Build history of the part. All positions in model axes, mm. Face numbers are marked on the shaded views. A direction names the side the tool comes from. Round coordinates to 2 decimals unless told otherwise and drop trailing zeros. Write each loop counter-clockwise with the first axis right and the second up, starting at its lowest first coordinate (ties: lowest second). Pieces come first, ordered by that corner, then holes. Notation, with made-up numbers: (66.25, 29) -> (123.25, 29) arc R33 ccw to (123.25, 68) -> close; hole circle Ø6 at (73.25, -26.75). An arc over 180 degrees is marked (long way). One line per question, with ' | ' between items.
from build123d import *

# Parameters (mm, degrees)
SKETCH1_W           = 60
SKETCH1_H           = 25
BOSS_EXTRUDE1_DEPTH = 1
SKETCH2_W           = 60
SKETCH2_H           = 25
SKETCH2_W_2         = 58
SKETCH2_H_2         = 23
BOSS_EXTRUDE2_DEPTH = 75
FILLET2_R           = 4
SKETCH4_R           = 7.5
SKETCH4_R_2         = 3.1
BOSS_EXTRUDE3_DEPTH = 10
FILLET3_R           = 5
SKETCH18_R          = 2
CUT_EXTRUDE6_DEPTH  = 1
SKETCH5_R           = 2.25
CUT_EXTRUDE1_DEPTH  = 98.63324229
SKETCH10_W          = 22.476776695
SKETCH10_H          = 22.501776695
BOSS_EXTRUDE4_DEPTH = 6
SKETCH12_W          = 2.5
SKETCH12_H          = 4.858493649
BOSS_EXTRUDE5_DEPTH = 15
SKETCH13_R          = 1.35
CUT_EXTRUDE3_DEPTH  = 12
SKETCH19_W          = 42
SKETCH19_H          = 66
CUT_EXTRUDE7_DEPTH  = 1
BOSS_EXTRUDE7_DEPTH = 2.5


with BuildPart() as part:
    # Sketch1 → Boss-Extrude1 (new body)
    with BuildSketch(Plane.XY):
        Rectangle(SKETCH1_W, SKETCH1_H)
    extrude(amount=-BOSS_EXTRUDE1_DEPTH)

    # Sketch2 → Boss-Extrude2 (add)
    with BuildSketch(Plane(origin=(0, 0, -1), x_dir=(-1, 0, 0), z_dir=(0, 0, -1))):
        Rectangle(SKETCH2_W, SKETCH2_H)
        Rectangle(SKETCH2_W_2, SKETCH2_H_2, mode=Mode.SUBTRACT)
    extrude(amount=BOSS_EXTRUDE2_DEPTH)

    # Fillet2
    fillet2_edges = [part.edges().sort_by_distance(p)[0] for p in [
        (-29, 11.5, -38.5),
        (29, 11.5, -38.5),
        (29, -11.5, -38.5),
        (-29, -11.5, -38.5),
        (30, -12.5, -38),
        (-30, -12.5, -38),
        (-30, 12.5, -38),
        (30, 12.5, -38),
    ]]
    fillet(fillet2_edges, radius=FILLET2_R)

    # Sketch4 → Boss-Extrude3 (add)
    # profile 1 of 2: a face of its own
    with BuildSketch(Plane.XY):
        with Locations((-17.5, 0)):
            Circle(SKETCH4_R)
        with Locations((-17.5, 0)):
            Circle(SKETCH4_R_2, mode=Mode.SUBTRACT)
    # profile 2 of 2: a face of its own
    with BuildSketch(Plane.XY):
        with Locations((17.5, 0)):
            Circle(SKETCH4_R)
        with Locations((17.5, 0)):
            Circle(SKETCH4_R_2, mode=Mode.SUBTRACT)
    extrude(amount=BOSS_EXTRUDE3_DEPTH)

    # Fillet3
    # the kernel refuses this fillet: 5 mm, written as the material it adds along each edge
    with BuildSketch(Plane(origin=(17.5, 0, 0), x_dir=(1, 0, 0), z_dir=(0, -1, 0))) as fillet3_piece_1:
        with BuildLine():
            CenterArc((7.5 + FILLET3_R, FILLET3_R), FILLET3_R, 180, 90)
            Line((7.5, FILLET3_R), (7.5, 0))
            Line((7.5, 0), (7.5 + FILLET3_R, 0))
        make_face()
    revolve(axis=Axis((17.5, 0, 0), (0, 0, 1)))
    with BuildSketch(Plane(origin=(-17.5, 0, 0), x_dir=(1, 0, 0), z_dir=(0, -1, 0))) as fillet3_piece_2:
        with BuildLine():
            CenterArc((7.5 + FILLET3_R, FILLET3_R), FILLET3_R, 180, 90)
            Line((7.5, FILLET3_R), (7.5, 0))
            Line((7.5, 0), (7.5 + FILLET3_R, 0))
        make_face()
    revolve(axis=Axis((-17.5, 0, 0), (0, 0, 1)))
    # the kernel refuses this fillet: 5 mm, written as the material it takes off along each edge
    with BuildSketch(Plane(origin=(17.5, 0, 10), x_dir=(1, 0, 0), z_dir=(0, -1, 0))) as fillet3_2_piece_1:
        with BuildLine():
            CenterArc((2.5, -4.963869458), FILLET3_R, 0, 83.107897421)
            Line((3.1, 0), (7.5, 0))
            Line((7.5, 0), (7.5, -4.963869458))
        make_face()
    revolve(axis=Axis((17.5, 0, 10), (0, 0, 1)), mode=Mode.SUBTRACT)
    with BuildSketch(Plane(origin=(-17.5, 0, 10), x_dir=(1, 0, 0), z_dir=(0, -1, 0))) as fillet3_2_piece_2:
        with BuildLine():
            CenterArc((2.5, -4.963869458), FILLET3_R, 0, 83.107897421)
            Line((3.1, 0), (7.5, 0))
            Line((7.5, 0), (7.5, -4.963869458))
        make_face()
    revolve(axis=Axis((-17.5, 0, 10), (0, 0, 1)), mode=Mode.SUBTRACT)

    # Sketch18 → Cut-Extrude6 (cut)
    with BuildSketch(Plane.XY):
        with Locations((-17.5, 0)):
            Circle(SKETCH18_R)
        with Locations((17.5, 0)):
            Circle(SKETCH18_R)
    extrude(amount=-CUT_EXTRUDE6_DEPTH, mode=Mode.SUBTRACT)

    # Sketch5 → Cut-Extrude1 (cut, through all)
    with BuildSketch(Plane(origin=(30, 0, 0), x_dir=(0, 0, -1), z_dir=(1, 0, 0))):
        with Locations((15, 0)):
            Circle(SKETCH5_R)
    extrude(amount=-CUT_EXTRUDE1_DEPTH, mode=Mode.SUBTRACT)

    # Sketch10 → Boss-Extrude4 (add)
    with BuildSketch(Plane(origin=(0, -11.5, 0), x_dir=(1, 0, 0), z_dir=(0, 1, 0))):
        with Locations((7.241611652, 35.500888348)):
            Rectangle(SKETCH10_W, SKETCH10_H)
    extrude(amount=BOSS_EXTRUDE4_DEPTH)

    # Sketch12 → Boss-Extrude5 (add)
    with BuildSketch(Plane(origin=(0, -11.5, 0), x_dir=(1, 0, 0), z_dir=(0, 1, 0))):
        with Locations((12.08, 21.824246825)):
            Rectangle(SKETCH12_W, SKETCH12_H)
        with Locations((12.08, 49.165753176)):
            Rectangle(SKETCH12_W, SKETCH12_H)
    extrude(amount=BOSS_EXTRUDE5_DEPTH)

    # Sketch13 → Cut-Extrude3 (cut)
    with BuildSketch(Plane(origin=(13.33, 0, 0), x_dir=(0, 0, -1), z_dir=(1, 0, 0))):
        with Locations((21.82424682, 0)):
            Circle(SKETCH13_R)
        with Locations((49.165753171, 0)):
            Circle(SKETCH13_R)
    extrude(amount=-CUT_EXTRUDE3_DEPTH, mode=Mode.SUBTRACT)

    # Sketch19 → Cut-Extrude7 (cut)
    with BuildSketch(Plane(origin=(0, 12.5, 0), x_dir=(1, 0, 0), z_dir=(0, 1, 0))):
        with Locations((0, 38)):
            Rectangle(SKETCH19_W, SKETCH19_H)
    extrude(amount=-CUT_EXTRUDE7_DEPTH, mode=Mode.SUBTRACT)

    # Sketch20 → Boss-Extrude7 (add)
    with BuildSketch(Plane(origin=(0, 0, -76), x_dir=(-1, 0, 0), z_dir=(0, 0, -1))):
        with BuildLine():
            Line((-25, 11.5), (25, 11.5))
            ThreePointArc((25, 11.5), (27.828427125, 10.328427125), (29, 7.5))
            Line((29, 7.5), (29, -7.5))
            ThreePointArc((29, -7.5), (27.828427125, -10.328427125), (25, -11.5))
            Line((25, -11.5), (-25, -11.5))
            ThreePointArc((-25, -11.5), (-27.828427125, -10.328427125), (-29, -7.5))
            Line((-29, -7.5), (-29, 7.5))
            ThreePointArc((-29, 7.5), (-27.828427125, 10.328427125), (-25, 11.5))
        make_face()
    extrude(amount=-BOSS_EXTRUDE7_DEPTH)


solid = part.part
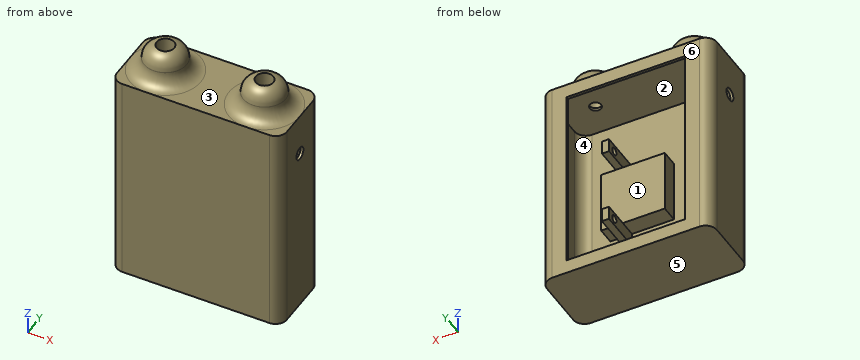
(1) 3-axis set-ups, long thin cutter, end or side, ignore diameter. For the marked faces 1, 2 and 3: which of +Z, -Z, +X, -X, +Y, -Y reach the whole face in a straight line?
Calculated:
face 1: +Y | face 2: none | face 3: +Z
(2) Slice it at B-B (x = -3). Write the cut outline in (y, z), then the cut area to 3 significant figures.
Calculated:
outline: (-12.5, -76) -> (12.5, -76) -> (12.5, -71) -> (11.5, -71) -> (11.5, -73.5) -> (-11.5, -73.5) -> (-11.5, -46.75) -> (-5.5, -46.75) -> (-5.5, -24.25) -> (-11.5, -24.25) -> (-11.5, -1) -> (11.5, -1) -> (11.5, -5) -> (12.5, -5) -> (12.5, 0) -> (-12.5, 0) -> close | area: 302 mm2
(3) Slice it at C-C (z = -61). Write the cut outline in (x, y), then the cut area to 3 significant figures.
Calculated:
outline: (-30, -8.5) arc R4 ccw to (-26, -12.5) -> (26, -12.5) arc R4 ccw to (30, -8.5) -> (30, 8.5) arc R4 ccw to (26, 12.5) -> (21, 12.5) -> (21, 11.5) -> (25, 11.5) arc R4 cw to (29, 7.5) -> (29, -7.5) arc R4 cw to (25, -11.5) -> (-25, -11.5) arc R4 cw to (-29, -7.5) -> (-29, 7.5) arc R4 cw to (-25, 11.5) -> (-21, 11.5) -> (-21, 12.5) -> (-26, 12.5) arc R4 ccw to (-30, 8.5) -> close | area: 124 mm2
(4) Slice it at D-D (z = 3.5). Write the cut outline in (x, y), then the cut area to 3 significant figures.
Calculated:
outline: circle Ø15.46 at (-17.5, 0); circle Ø15.46 at (17.5, 0); hole circle Ø6.2 at (-17.5, 0); hole circle Ø6.2 at (17.5, 0) | area: 315 mm2
(5) Mould opens along Y. For the marked faces 4, 5 and 6 say: pulls with the +Y half, pulls with the -Y half, needs draft (parallel to the pull), parting line crosses it, or undercut.
Calculated:
face 4: undercut | face 5: needs draft | face 6: pulls with the +Y half
(6) Slice it at A-A (z = -15). Write the cut outline in (x, y).
Calculated:
outline: (-30, -8.5) arc R4 ccw to (-26, -12.5) -> (26, -12.5) arc R4 ccw to (30, -8.5) -> (30, -2.25) -> (29, -2.25) -> (29, -7.5) arc R4 cw to (25, -11.5) -> (-25, -11.5) arc R4 cw to (-29, -7.5) -> (-29, -2.25) -> (-30, -2.25) -> close; (-30, 2.25) -> (-29, 2.25) -> (-29, 7.5) arc R4 cw to (-25, 11.5) -> (-21, 11.5) -> (-21, 12.5) -> (-26, 12.5) arc R4 ccw to (-30, 8.5) -> close; (21, 11.5) -> (25, 11.5) arc R4 cw to (29, 7.5) -> (29, 2.25) -> (30, 2.25) -> (30, 8.5) arc R4 ccw to (26, 12.5) -> (21, 12.5) -> close
(7) Drop flat-ended pins along their axis: pin 1 (0.8 mm diameter, centred on x = 12.5, y = -5.5, fed in from +Z); pin 2 (2 mm diameter, centred on x = 18.5, z = -25.5, fed in from +Y); pin 3 (6.5 mm diameter, centred on x = 6.5, y = -8.5, fed in from +Z). Give the stop position or say it passes through.
Calculated:
pin 1: z = 7.15 | pin 2: y = -5.5 | pin 3: z = 0.35
(8) Wall check: line 1 (X direction, y = 1.5, z = -22.5); line 2 (X direction, y = 3.25, z = -35); line 3 (Y direction, x = 23, z = -39). Give the ranges that are in metal, low to high. Write a range as from..to.
Calculated:
line 1: -30..-29, 10.83..13.33, 29..30 | line 2: -30..-29, 29..30 | line 3: -12.5..-11.5, 11.5..12.5
